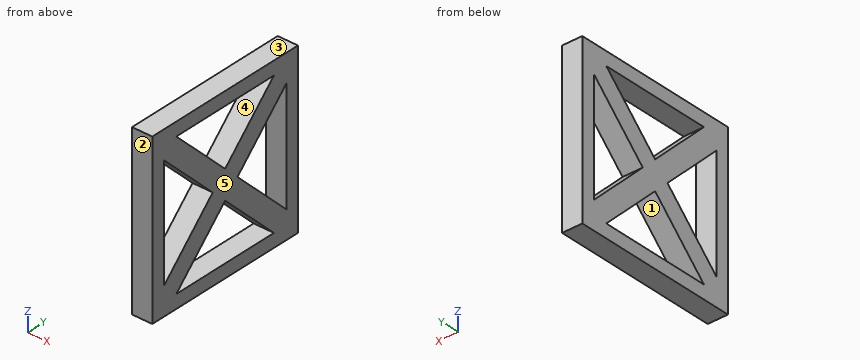
from build123d import *

# Parameters (mm, degrees)
SKETCH1_W           = 50
SKETCH1_H           = 50
BOSS_EXTRUDE1_DEPTH = 6


with BuildPart() as part:
    # Sketch1 → Boss-Extrude1 (new body)
    with BuildSketch(Plane.YZ):
        Rectangle(SKETCH1_W, SKETCH1_H)
        Polygon((4.242640687, 0), (21, 16.757359313), (21, -16.757359313), align=None, mode=Mode.SUBTRACT)
        Polygon((16.757359313, 21), (0, 4.242640687), (-16.757359313, 21), align=None, mode=Mode.SUBTRACT)
        Polygon((-21, 16.757359313), (-4.242640687, 0), (-21, -16.757359313), align=None, mode=Mode.SUBTRACT)
        Polygon((-16.757359313, -21), (0, -4.242640687), (16.757359313, -21), align=None, mode=Mode.SUBTRACT)
    extrude(amount=BOSS_EXTRUDE1_DEPTH)


solid = part.part
Verification items for the finished model (mm, model axes). Face numbers are marked on the shaded views. A direction names the side the tool comes from. Coordinates: 2 decimals unless noted, no trailing zeros. Loops run counter-clockwise (first coordinate to the right, second up) from the corner with the lowest first, then second, coordinate; pieces in that order, holes last. Notation, with made-up numbers: (77.5, 56.5) -> (118.5, 56.5) arc R21 cw to (118.5, 79.5) -> close; hole circle Ø11 at (55, -18.5). An arc over 180 degrees is marked (long way). Answer as a JSON object with one key per item and string values. Group by question number.
Item 1: Sectioned sample at D-D on y = 12. Record the boundary of the cut face in (x, z).
Item 2: Sectioned sample at B-B on z = -17.5. Record the boundary of the cut face in (x, y), plus the area to 3 significant figures.
Item 3: Sectioned sample at C-C on z = 5. Record the boundary of the cut face in (x, y).
Item 4: Sectioned sample at A-A on x = 3.8. Record the boundary of the cut face in (y, z).
Item 5: Tool access check on the marked faces 4 and 5. Record the directions out of +Z, -Z, +X, -X, +Y, -Y that give a thin tool (end or side, any length) a straight path to the whole face; none if there is none.
Item 6: Mould release check, pull along Y, two halves, no side actions. Record for the marked faces 1, 2 and 3: +Y half, -Y half, draft (parallel to the pull), parting line (faces both ways), or undercut.
Item 7: Scan lines: probe 1 along Z at (x, y) = (2.75, -7); probe 2 along Z at (x, y) = (3.1, -10); probe 3 along Z at (x, y) = (1.1, 1). Record each from-to range of solid material in increasing order.
Evaluation:
{
 "1": {"outline": "(0, -25) -> (6, -25) -> (6, -21) -> (0, -21) -> close; (0, -16.24) -> (6, -16.24) -> (6, -7.76) -> (0, -7.76) -> close; (0, 7.76) -> (6, 7.76) -> (6, 16.24) -> (0, 16.24) -> close; (0, 21) -> (6, 21) -> (6, 25) -> (0, 25) -> close"},
 "2": {"outline": "(0, -25) -> (6, -25) -> (6, -13.26) -> (0, -13.26) -> close; (0, 13.26) -> (6, 13.26) -> (6, 25) -> (0, 25) -> close", "area": "141 mm²"},
 "3": {"outline": "(0, -25) -> (6, -25) -> (6, -21) -> (0, -21) -> close; (0, -9.24) -> (6, -9.24) -> (6, -0.76) -> (0, -0.76) -> close; (0, 0.76) -> (6, 0.76) -> (6, 9.24) -> (0, 9.24) -> close; (0, 21) -> (6, 21) -> (6, 25) -> (0, 25) -> close"},
 "4": {"outline": "(-25, -25) -> (25, -25) -> (25, 25) -> (-25, 25) -> close; hole (-21, -16.76) -> (-4.24, 0) -> (-21, 16.76) -> close; hole (-16.76, -21) -> (16.76, -21) -> (0, -4.24) -> close; hole (-16.76, 21) -> (0, 4.24) -> (16.76, 21) -> close; hole (4.24, 0) -> (21, -16.76) -> (21, 16.76) -> close"},
 "5": {"face 4": "+X, -X", "face 5": "+Z, -Z, +X, +Y, -Y"},
 "6": {"face 1": "undercut", "face 2": "-Y half", "face 3": "draft"},
 "7": {"probe 1": "z = -25 to -21, -11.24 to -2.76, 2.76 to 11.24, 21 to 25", "probe 2": "z = -25 to -21, -14.24 to -5.76, 5.76 to 14.24, 21 to 25", "probe 3": "z = -25 to -21, -5.24 to 5.24, 21 to 25"}
}
